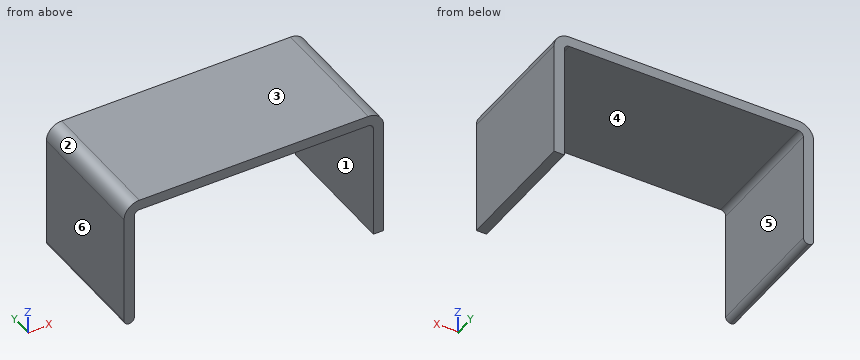
```python
from build123d import *

# Parameters (mm, degrees)
F0_W     = 50.8
F0_H     = 25.4
F1_DEPTH = 12.7
F2_W     = 46.8
F2_H     = 23.4
F3_DEPTH = 25.4
F4_R     = 3
F5_R     = 1
F6_R     = 0.99999


# Not quite as in the source:
# - a fillet or chamfer is up to 0.001 mm smaller than in the source, because OpenCascade refuses the exact size


with BuildPart() as f1:
    # F0 (on Front) → F1 (new body, symmetric)
    with BuildSketch(Plane.XZ):
        Rectangle(F0_W, F0_H)
    extrude(amount=F1_DEPTH, both=True)

    # F2 (on face) → F3 (cut, through all)
    with BuildSketch(Plane.XZ.offset(12.7)):
        with Locations((0, -1)):
            Rectangle(F2_W, F2_H)
    extrude(amount=-F3_DEPTH, mode=Mode.SUBTRACT)

    # F4
    f4_edges = [f1.edges().sort_by_distance(p)[0] for p in [
        (-25.4, 0, 12.7),
        (25.4, 0, 12.7),
    ]]
    fillet(f4_edges, radius=F4_R)

    # F5
    f5_edges = [f1.edges().sort_by_distance(p)[0] for p in [
        (-23.4, 0, 10.7),
        (23.4, 0, 10.7),
    ]]
    fillet(f5_edges, radius=F5_R)

    # F6 (radius 1 in the source; OpenCascade refuses exactly that, so slightly less here)
    f6_edges = [f1.edges().sort_by_distance(p)[0] for p in [
        (-25.4, 0, -12.7),
        (-23.4, 0, -12.7),
    ]]
    fillet(f6_edges, radius=F6_R)


solid = f1.part
```
Verification items for the finished model (mm, model axes). Face numbers are marked on the shaded views. A direction names the side the tool comes from. Coordinates: 2 decimals unless noted, no trailing zeros. Write each loop counter-clockwise with the first axis right and the second up, starting at its lowest first coordinate (ties: lowest second). Pieces come first, ordered by that corner, then holes. Notation, with made-up numbers: (25.5, 85.5) - (68.5, 85.5) arc R22 ccw to (68.5, 108.5) - close; hole circle Ø10 at (45, 36.25). An arc over 180 degrees is marked (long way). One line per question, with ' | ' between items. Start each with the question number.
1. Material ranges on line 1 along X through (y, z) = (-10.25, -7.5); line 2 along Z through (x, y) = (-18, 8.75); line 3 along X through (y, z) = (-6, 10.5), recorded low to high.
2. Gauge pin test, flat end, axial feed: P1, Ø1.5, axis at x = -0.5, y = -4.5, coming from the -Z side. Record the tip position at first contact, or that the pin passes through.
3. Draft check along X on the marked faces 3, 4, 5 and 6. Enter one of: released by +X, released by -X, zero draft, split by the parting line, or undercut.
4. Access from +Z, -Z, +X, -X, +Y, -Y to the whole of each face (thin tool, end or side, straight path). Record for the marked faces 1 and 2.
5. Section check A-A (z = -5.25). Enter the section's corners in (x, y), plus the area to 3 significant figures.
6. Section check C-C (x = -6). Enter the section's corners in (y, z), plus the area to 3 significant figures.
Computed values:
1) line 1: -25.4 to -23.4, 23.4 to 25.4 | line 2: 10.7 to 12.7 | line 3: -25.29 to -23, 23 to 25.29
2) P1: z = 10.7
3) face 3: zero draft | face 4: undercut | face 5: undercut | face 6: released by -X
4) face 1: -Z, +Y, -Y | face 2: +Z, -X, +Y, -Y
5) outline: (-25.4, -12.7) - (-23.4, -12.7) - (-23.4, 12.7) - (-25.4, 12.7) - close; (23.4, -12.7) - (25.4, -12.7) - (25.4, 12.7) - (23.4, 12.7) - close | area: 102 mm²
6) outline: (-12.7, 10.7) - (12.7, 10.7) - (12.7, 12.7) - (-12.7, 12.7) - close | area: 50.8 mm²
